For this review, take the finished solid that the model builds, in its own axes (mm). A direction names the side the tool comes from. Round coordinates to 2 decimals unless told otherwise and drop trailing zeros. Order: outer loops, then holes, each group sorted by start corner. A loop starts at its lowest first (then second) coordinate and runs counter-clockwise, first axis right, second up. Notation, with made-up numbers: M 49,51.5 L 99,51.5 A23 cw 99,72.5 Z; hole C -3,-29 d6. An arc over 180 degrees is marked long. Use a Markdown table: item, result.
Autodesk Inventor part; units mm, degrees
ref_plane "YZ Plane" through (0, 0, 0) normal (1, 0, 0) x (0, 1, 0)
ref_plane "XZ Plane" through (0, 0, 0) normal (0, 1, 0) x (-1, 0, 0)
ref_plane "XY Plane" through (0, 0, 0) normal (0, 0, 1) x (1, 0, 0)
sketch "Эскиз1" plane through (0, 0, 0) normal (0, 1, 0) x (-1, 0, 0)
  line L0 (9.374, 18.1547) -> (1.5, 18.1547)
  line L1 (1.5, 18.1547) -> (1.5, 15.4147)
  line L2 (1.5, 15.4147) -> (9.374, 15.4147)
  line L3 (9.374, 15.4147) -> (9.374, 18.1547)
  line L4 (9.374, 7.9747) -> (1.5, 7.9747)
  line L5 (1.5, 7.9747) -> (1.5, 4.9747)
  line L6 (1.5, 4.9747) -> (9.374, 4.9747)
  line L7 (9.374, 4.9747) -> (9.374, 7.9747)
  line L8 (10.2755, 20.6947) -> (0, 20.6947)
  line L9 (0, 20.6947) -> (0, 3.6947)
  line L10 (0, 3.6947) -> (10.2755, 3.6947)
  line L11 (10.2755, 3.6947) -> (10.2755, 20.6947)
  point P0 (0, 0)
  dimension "d3" = 17
  dimension "d4" = 7.874
  dimension "d5" = 2.74
  dimension "d6" = 2.54
  dimension "d7" = 7.44
  dimension "d8" = 1.5
  dimension "d11" = 3
extrude "Выдавливание1" add sketch "Эскиз1" along normal blind 2
sketch "Эскиз3" plane through (0, 0, 0) normal (0, -1, 0) x (1, 0, 0)
  line L0 (-8.9898, 13.0238) -> (-0.8671, 13.0238) construction
  line L1 (-0.8671, 13.0238) -> (-0.8671, 9.5038) construction
  line L2 (-0.8671, 9.5038) -> (-8.9898, 9.5038) construction
  line L3 (-8.9898, 9.5038) -> (-8.9898, 13.0238) construction
  spline S0 degree 2 poles (-7.8313, 9.8672) (-8.1623, 9.8672) (-8.6267, 10.0055) (-8.8317, 10.1043) knots 0 0 0 1 2 2 2
  line L4 (-8.8317, 10.1043) -> (-8.8317, 10.6131)
  line L5 (-8.8317, 10.6131) -> (-8.802, 10.6131)
  spline S1 degree 2 poles (-8.802, 10.6131) (-8.602, 10.4254) (-8.0956, 10.2179) (-7.861, 10.2179) knots 0 0 0 1 2 2 2
  spline S2 degree 2 poles (-7.861, 10.2179) (-7.525, 10.2179) (-7.1817, 10.497) (-7.1817, 10.7267) knots 0 0 0 1 2 2 2
  spline S3 degree 2 poles (-7.1817, 10.7267) (-7.1817, 10.9095) (-7.362, 11.1367) (-7.5572, 11.1936) knots 0 0 0 1 2 2 2
  spline S4 degree 2 poles (-7.5572, 11.1936) (-7.6979, 11.2331) (-7.9326, 11.2874) (-8.108, 11.3319) knots 0 0 0 1 2 2 2
  spline S5 degree 2 poles (-8.108, 11.3319) (-8.2661, 11.3739) (-8.5155, 11.4998) (-8.6119, 11.6011) knots 0 0 0 1 2 2 2
  spline S6 degree 2 poles (-8.6119, 11.6011) (-8.7057, 11.7024) (-8.8095, 11.9741) (-8.8095, 12.1519) knots 0 0 0 1 2 2 2
  spline S7 degree 2 poles (-8.8095, 12.1519) (-8.8095, 12.5224) (-8.2315, 13.0238) (-7.7844, 13.0238) knots 0 0 0 1 2 2 2
  spline S8 degree 2 poles (-7.7844, 13.0238) (-7.5275, 13.0238) (-7.073, 12.9226) (-6.8779, 12.8262) knots 0 0 0 1 2 2 2
  line L6 (-6.8779, 12.8262) -> (-6.8779, 12.3421)
  line L7 (-6.8779, 12.3421) -> (-6.9075, 12.3421)
  spline S9 degree 2 poles (-6.9075, 12.3421) (-7.0533, 12.4755) (-7.5078, 12.6731) (-7.7572, 12.6731) knots 0 0 0 1 2 2 2
  spline S10 degree 2 poles (-7.7572, 12.6731) (-8.0388, 12.6731) (-8.3871, 12.4088) (-8.3871, 12.1939) knots 0 0 0 1 2 2 2
  spline S11 degree 2 poles (-8.3871, 12.1939) (-8.3871, 12.0012) (-8.1821, 11.7715) (-7.9894, 11.7197) knots 0 0 0 1 2 2 2
  spline S12 degree 2 poles (-7.9894, 11.7197) (-7.861, 11.6851) (-7.488, 11.5962) (-7.3645, 11.5591) knots 0 0 0 1 2 2 2
  spline S13 degree 2 poles (-7.3645, 11.5591) (-7.0508, 11.4628) (-6.7593, 11.075) (-6.7593, 10.7909) knots 0 0 0 1 2 2 2
  spline S14 degree 2 poles (-6.7593, 10.7909) (-6.7593, 10.6106) (-6.9051, 10.2648) (-7.036, 10.1438) knots 0 0 0 1 2 2 2
  spline S15 degree 2 poles (-7.036, 10.1438) (-7.1817, 10.0104) (-7.5522, 9.8672) (-7.8313, 9.8672) knots 0 0 0 1 2 2 2
  line L8 (-4.1362, 12.9695) -> (-5.1859, 9.9215)
  line L9 (-5.1859, 9.9215) -> (-5.6231, 9.9215)
  line L10 (-5.6231, 9.9215) -> (-6.6729, 12.9695)
  line L11 (-6.6729, 12.9695) -> (-6.2382, 12.9695)
  line L12 (-6.2382, 12.9695) -> (-5.3934, 10.4377)
  line L13 (-5.3934, 10.4377) -> (-4.5487, 12.9695)
  line L14 (-4.5487, 12.9695) -> (-4.1362, 12.9695)
  spline S16 degree 2 poles (-2.5677, 9.8622) (-2.8913, 9.8622) (-3.4273, 10.0598) (-3.62, 10.2599) knots 0 0 0 1 2 2 2
  spline S17 degree 2 poles (-3.62, 10.2599) (-3.8126, 10.4624) (-4.0176, 11.0602) (-4.0176, 11.448) knots 0 0 0 1 2 2 2
  spline S18 degree 2 poles (-4.0176, 11.448) (-4.0176, 11.816) (-3.8101, 12.3989) (-3.6175, 12.6064) knots 0 0 0 1 2 2 2
  spline S19 degree 2 poles (-3.6175, 12.6064) (-3.4322, 12.8065) (-2.8888, 13.0238) (-2.5653, 13.0238) knots 0 0 0 1 2 2 2
  spline S20 degree 2 poles (-2.5653, 13.0238) (-2.4096, 13.0238) (-2.1281, 12.9794) (-1.9996, 12.9399) knots 0 0 0 1 2 2 2
  spline S21 degree 2 poles (-1.9996, 12.9399) (-1.8959, 12.9102) (-1.6439, 12.8015) (-1.5674, 12.762) knots 0 0 0 1 2 2 2
  line L15 (-1.5674, 12.762) -> (-1.5674, 12.2729)
  line L16 (-1.5674, 12.2729) -> (-1.6019, 12.2729)
  spline S22 degree 2 poles (-1.6019, 12.2729) (-1.6785, 12.3396) (-1.8391, 12.4607) (-1.9873, 12.5298) knots 0 0 0 1 2 2 2
  spline S23 degree 2 poles (-1.9873, 12.5298) (-2.1108, 12.5916) (-2.4294, 12.6731) (-2.6122, 12.6731) knots 0 0 0 1 2 2 2
  spline S24 degree 2 poles (-2.6122, 12.6731) (-3.0518, 12.6731) (-3.5953, 12.0111) (-3.5953, 11.4603) knots 0 0 0 1 2 2 2
  spline S25 degree 2 poles (-3.5953, 11.4603) (-3.5953, 11.154) (-3.452, 10.6946) (-3.3161, 10.5365) knots 0 0 0 1 2 2 2
  spline S26 degree 2 poles (-3.3161, 10.5365) (-3.1852, 10.3784) (-2.8147, 10.213) (-2.5825, 10.213) knots 0 0 0 1 2 2 2
  spline S27 degree 2 poles (-2.5825, 10.213) (-2.4121, 10.213) (-2.0713, 10.2624) (-1.9552, 10.3118) knots 0 0 0 1 2 2 2
  line L17 (-1.9552, 10.3118) -> (-1.9552, 11.0997)
  line L18 (-1.9552, 11.0997) -> (-2.6616, 11.0997)
  line L19 (-2.6616, 11.0997) -> (-2.6616, 11.4554)
  line L20 (-2.6616, 11.4554) -> (-1.555, 11.4554)
  line L21 (-1.555, 11.4554) -> (-1.555, 10.124)
  spline S28 degree 2 poles (-1.555, 10.124) (-1.6316, 10.0895) (-1.8934, 9.9832) (-2.0046, 9.9511) knots 0 0 0 1 2 2 2
  spline S29 degree 2 poles (-2.0046, 9.9511) (-2.1552, 9.9067) (-2.3973, 9.8622) (-2.5677, 9.8622) knots 0 0 0 1 2 2 2
  point P0 (0, 0)
extrude "Выдавливание2" cut sketch "Эскиз3" against normal blind 0.4
properties part number "подшипник_крепеж"
Q1. Draft analysis for pull direction X (two halves, no side actions). For faces 1 (the flat face through (-1.5, 1, 6)), 2 (the flat face through (-10.276, 1, 12)), 3 (the flat face through (-4.654, 0.197, 11.467)), 4 (the flat face through (-5, 1, 20.695)), state which applies: pulls with the +X half, pulls with the -X half, needs draft (parallel to the pull), parting line crosses it, or undercut.
Determined:
| item | result |
|---|---|
| face 1 | undercut |
| face 2 | pulls with the -X half |
| face 3 | undercut |
| face 4 | needs draft |
Q2. Add section B-B (z = 7). Write out the cut boundary in (x, y), then the cut area to 3 significant figures.
Determined:
| item | result |
|---|---|
| outline | M -10.28,0 L -9.37,0 L -9.37,2 L -10.28,2 Z; M -1.5,0 L 0,0 L 0,2 L -1.5,2 Z |
| area | 4.80 mm^2 |
Q3. Add section C-C (x = -4.75). Write out the cut boundary in (y, z).
Determined:
| item | result |
|---|---|
| outline | M 0,3.69 L 2,3.69 L 2,4.97 L 0,4.97 Z; M 0,7.97 L 2,7.97 L 2,15.41 L 0,15.41 L 0,12.37 L 0.4,12.37 L 0.4,11.19 L 0,11.19 Z; M 0,18.15 L 2,18.15 L 2,20.69 L 0,20.69 Z |
Q4. Wall thickness on line 1 along Z through (x, y) = (-9, 1.6); line 2 along X through (y, z) = (0.2, 16.5); line 3 along Z through (x, y) = (-8.25, 0.35): over which ranges is each line inside the solid? List them lowest first. Write a range as [from, to].
Determined:
| item | result |
|---|---|
| line 1 | z = [3.69, 4.97], [7.97, 15.41], [18.15, 20.69] |
| line 2 | x = [-10.28, -9.37], [-1.5, 0] |
| line 3 | z = [3.69, 4.97], [7.97, 9.9], [10.28, 11.38], [11.85, 12.51], [12.94, 15.41], [18.15, 20.69] |
Q5. Add section D-D (x = -3). Give the number of separate pieces and of enclosed holes in the cut face, then the cut area to 3 significant figures.
Determined:
| item | result |
|---|---|
| separate pieces | 3 |
| enclosed holes | 0 |
| area | 22.2 mm^2 |
Q6. Add section A-A (y = 1.35). Write out the cut boundary in (x, z), then the cut area to 3 significant figures.
Determined:
| item | result |
|---|---|
| outline | M -10.28,3.69 L 0,3.69 L 0,20.69 L -10.28,20.69 Z; hole M -9.37,4.97 L -1.5,4.97 L -1.5,7.97 L -9.37,7.97 Z; hole M -9.37,15.41 L -1.5,15.41 L -1.5,18.15 L -9.37,18.15 Z |
| area | 129 mm^2 |
Q7. Machinability: for faces 5 (the flat face through (-6.14, 0.2, 11.42)), 6 (the flat face through (-5, 1, 4.975)), 7 (the flat face through (-5, 2, 12)), which of the approach directions +Z, -Z, +X, -X, +Y, -Y give a long, thin tool a straight path to every point of the face, cutting with its end or side? Answer none if there is none.
Determined:
| item | result |
|---|---|
| face 5 | -Y |
| face 6 | +Y, -Y |
| face 7 | +Z, -Z, +X, -X, +Y |
